Input: part model. Units: mm. Frame: model coordinates. Face numbers are marked on the shaded views. A direction names the side the tool comes from. Give positions to 0.01 mm unless a question says otherwise; leave off trailing zeros. Loops run counter-clockwise (first coordinate to the right, second up) from the corner with the lowest first, then second, coordinate; pieces in that order, holes last. Notation, with made-up numbers: M 29.25,-1.5 L 37.25,-1.5 A26 ccw 37.25,34.5 Z; hole C -27,73.5 d10. An arc over 180 degrees is marked long. Answer as a JSON object with one key per item and string values. Group by question number.
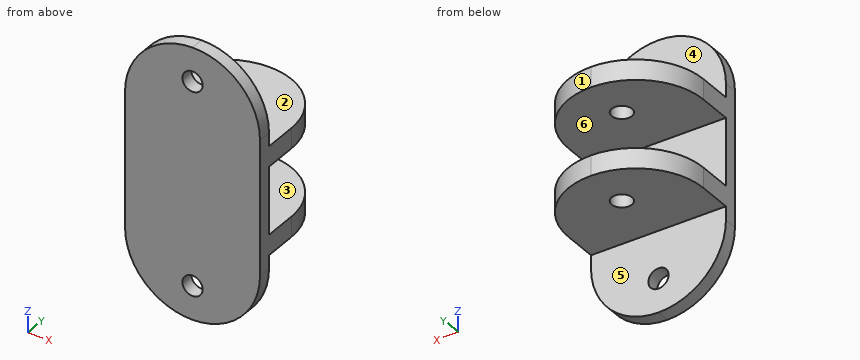
Autodesk Inventor part; units mm, degrees
ref_plane "YZ Plane" through (0, 0, 0) normal (1, 0, 0) x (0, 1, 0)
ref_plane "XZ Plane" through (0, 0, 0) normal (0, 1, 0) x (-1, 0, 0)
ref_plane "XY Plane" through (0, 0, 0) normal (0, 0, 1) x (1, 0, 0)
sketch "Sketch1" plane through (0, 0, 0) normal (0, 1, 0) x (-1, 0, 0)
  line L0 (-10, -20) -> (10, -20)
  line L1 (10, -20) -> (10, 20)
  line L2 (10, 20) -> (-10, 20)
  line L3 (-10, 20) -> (-10, -20)
  line L4 (-10, -20) -> (10, 20) construction
  line L5 (10, -20) -> (-10, 20) construction
  point P0 (0, 0)
  dimension "d0" = 20
  dimension "d1" = 40
extrude "Extrusion1" add sketch "Sketch1" along normal blind 2
sketch "Sketch3" plane through (0, 2, 0) normal (0, 1, 0) x (1, 0, 0)
  line L0 (-10, 20) -> (-10, -20)
  line L1 (10, -20) -> (10, 20)
  line L2 (-10, -8) -> (10, -8)
  line L3 (10, -8) -> (10, -5)
  line L4 (10, -5) -> (-10, -5)
  line L5 (-10, -5) -> (-10, -8)
  line L6 (-6.0097, 0) -> (5.0263, 0)
  line L7 (-10, 8) -> (10, 8)
  line L8 (10, 8) -> (10, 5)
  line L9 (10, 5) -> (-10, 5)
  line L10 (-10, 5) -> (-10, 8)
  point P0 (0, 0)
  dimension "d6" = 3
  dimension "d7" = 5
extrude "Extrusion2" add sketch "Sketch3" along normal blind 15 contours L7 L1 L9 L0 | L4 L1 L2 L0
fillet "Fillet1" radius 10 4 edges at (10, 17, 6.5) (-10, 17, 6.5) (10, 17, -6.5) (-10, 17, -6.5)
sketch "Sketch4" plane through (0, 2, 0) normal (0, 1, 0) x (1, 0, 0)
  line L0 (10, 20) -> (-10, 20)
  line L1 (-10, -20) -> (10, -20)
  point P0 (0, 0)
  point P1 (0, 15)
  point P2 (0, -15)
  dimension "d11" = 5
  dimension "d12" = 5
hole "Hole1" at (0, 2, -15) at (0, 2, 15) direction (0, -1, 0) diameter 3 end through all
fillet "Fillet2" radius 10 4 edges at (10, 1, 20) (-10, 1, 20) (-10, 1, -20) (10, 1, -20)
sketch "Sketch5" plane through (10, 2, -8) normal (0, 0, -1) x (-1, 0, 0)
  point P0 (10, -2)
  point P1 (10, 8.1411)
hole "Hole2" at (0, 10.1411, -8) direction (0, 0, 1) diameter 3 end through all
properties part number "turretSupport" material "PC/ABS Plastic"
1. Material intervals for L1, parallel to Z at x = 0, y = 0.55; L2, parallel to Y at x = 0, z = 6.6; L3, parallel to Z at x = 4, y = 15.25, sorted ascending.
2. Section C-C (x = -5.5). Output: boundary loops of the cut face in (y, z), then the cut area to 3 significant figures.
3. Section B-B (z = 15). Output: boundary loops of the cut face in (x, y), then the cut area to 3 significant figures.
4. Mould query, pull axis Z, two halves, no side actions, for the marked faces 1, 2 and 3. Classes: pulls with the +Z half, pulls with the -Z half, needs draft (parallel to the pull), parting line crosses it, or undercut.
5. Reachability of the marked faces 4, 5 and 6 from +Z, -Z, +X, -X, +Y, -Y: full face, straight path, thin tool, end or side. Return the list, or none.
6. First-contact query: P1, Ø1, axis at x = 6, z = -10, coming from the -Y side; P2, Ø1.5, axis at y = 3.5, z = -16, coming from the +X side; P3, Ø10, axis at x = 6, z = 8.5, coming from the +Y side; P4, Ø1.5, axis at x = 7, y = 15, coming from the -Z side. Flat tips, straight axial feed; report the tip coordinate or a pass-through.
7. Section A-A (y = 3.25). Output: boundary loops of the cut face in (x, z).
8. Section D-D (z = -0.5). Output: boundary loops of the cut face in (x, y), then the cut area to 3 significant figures.
Geometry results:
{
 "1": {"L1": "-20 to -16.5, -13.5 to 13.5, 16.5 to 20", "L2": "0 to 8.64, 11.64 to 17", "L3": "-8 to -5, 5 to 8"},
 "2": {"outline": "M 0,-18.35 L 2,-18.35 L 2,-8 L 15.35,-8 L 15.35,-5 L 2,-5 L 2,5 L 15.35,5 L 15.35,8 L 2,8 L 2,18.35 L 0,18.35 Z", "area": "154 mm2"},
 "3": {"outline": "M -8.66,0 L -1.5,0 L -1.5,2 L -8.66,2 Z; M 1.5,0 L 8.66,0 L 8.66,2 L 1.5,2 Z", "area": "28.6 mm2"},
 "4": {"face 1": "needs draft", "face 2": "pulls with the +Z half", "face 3": "undercut"},
 "5": {"face 4": "+Z, +X, -X, +Y", "face 5": "-Z, +X, -X, +Y", "face 6": "+X, -X, +Y"},
 "6": {"P1": "y = 0", "P2": "through", "P3": "y = 16.95", "P4": "z = -8"},
 "7": {"outline": "M -10,-8 L 10,-8 L 10,-5 L -10,-5 Z; M -10,5 L 10,5 L 10,8 L -10,8 Z"},
 "8": {"outline": "M -10,0 L 10,0 L 10,2 L -10,2 Z", "area": "40.0 mm2"}
}
